from build123d import *


with BuildPart() as part:
    # Sketch1 → Revolve1 (revolve)
    with BuildSketch(Plane(origin=(0, 0, 0), x_dir=(1, 0, 0), z_dir=(0, 1, 0))):
        with BuildLine():
            Line((-12, 8), (-2.5, 8))
            Line((-2.5, 8), (-2.5, 27))
            Line((-2.5, 27), (-12, 27))
            Line((-12, 27), (-12, 30))
            ThreePointArc((-12, 30), (0, 50), (12, 30))
            Line((12, 30), (12, 27))
            Line((12, 27), (2.5, 27))
            Line((2.5, 27), (2.5, 8))
            Line((2.5, 8), (12, 8))
            Line((12, 8), (12, 5))
            Line((12, 5), (-12, 5))
            Line((-12, 5), (-12, 8))
        make_face()
    revolve(axis=Axis((-7.022018073, 0, 0), (1, 0, 0)))


solid = part.part
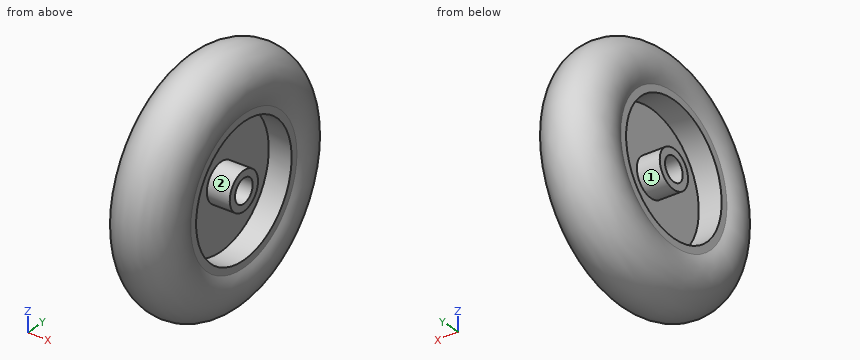
Could you check a few things on this model? Use its own coordinates, in mm. Face numbers are marked on the shaded views. A direction names the side the tool comes from. Coordinates: 2 decimals unless noted, no trailing zeros. Loops run counter-clockwise (first coordinate to the right, second up) from the corner with the lowest first, then second, coordinate; pieces in that order, holes last.
1. For the marked faces 1 and 2, which set-ups out of +Z, -Z, +X, -X, +Y, -Y let a thin tool reach every point of the face, with its end or its side?
2. For P1, Ø13, axis at y = -3, z = 1.5, coming from the -X side; P2, Ø3, axis at y = 19.5, z = -37, coming from the +X side; P3, Ø3, axis at x = 7, z = 28, coming from the -Y side, each with a flat end and sliding along its axis, tell me the tip position at first contact or that it passes through.
3. I need wall thicknesses on L1, parallel to Y at x = 6.75, z = 0; L2, parallel to Y at x = 6.5, z = 0; L3, parallel to Z at x = -7, y = 6. Which ranges of each line are inside material? Lowest first, please.
4. Imagine slicing it at D-D (x = 9). Please give me the cut outline in (y, z).
5. Imagine slicing it at A-A (y = 0). Please give me the cut outline in (x, z).
6. Imagine slicing it at C-C (x = -10.5). Please give me the cut outline in (y, z), and give its area (3 significant figures).
Computed values:
1. face 1: -X
1. face 2: +X
2. P1: stops at x = -12
2. P2: stops at x = 13.02
2. P3: stops at y = -40.49
3. L1: y = -48.21 to -27, -8 to -5, 5 to 8, 27 to 48.21
3. L2: y = -48.35 to -27, -8 to -5, 5 to 8, 27 to 48.35
3. L3: z = -47.68 to -26.32, -5.29 to 5.29, 26.32 to 47.68
4. outline: circle Ø93.19 at (0, 0); circle Ø16 at (0, 0); hole circle Ø54 at (0, 0); hole circle Ø10 at (0, 0)
5. outline: (-12, -30) arc R13.6 ccw (long way) to (12, -30) - (12, -27) - (2.5, -27) - (2.5, -8) - (12, -8) - (12, -5) - (-12, -5) - (-12, -8) - (-2.5, -8) - (-2.5, -27) - (-12, -27) - close; (-12, 5) - (12, 5) - (12, 8) - (2.5, 8) - (2.5, 27) - (12, 27) - (12, 30) arc R13.6 ccw (long way) to (-12, 30) - (-12, 27) - (-2.5, 27) - (-2.5, 8) - (-12, 8) - close
6. outline: circle Ø90.09 at (0, 0); circle Ø16 at (0, 0); hole circle Ø54 at (0, 0); hole circle Ø10 at (0, 0)
6. area: 4,210 mm2
